```python
from build123d import *

# Parameters (mm, degrees)
SKETCH1_W           = 20
SKETCH1_H           = 25
SKETCH1_R           = 1
SKETCH1_W_2         = 12
SKETCH1_H_2         = 15
BOSS_EXTRUDE1_DEPTH = 1.5


with BuildPart() as part:
    # Sketch1 → Boss-Extrude1 (new, symmetric)
    with BuildSketch(Plane(origin=(0, 0, 0), x_dir=(1, 0, 0), z_dir=(0, 1, 0))):
        Rectangle(SKETCH1_W, SKETCH1_H)
        with Locations(Location((-8, -2.5, 0), (0, 0, 270))):
            Circle(SKETCH1_R, mode=Mode.SUBTRACT)
        with Locations(Location((8, -2.5, 0), (0, 0, 90))):
            Circle(SKETCH1_R, mode=Mode.SUBTRACT)
        Rectangle(SKETCH1_W_2, SKETCH1_H_2, mode=Mode.SUBTRACT)
    extrude(amount=BOSS_EXTRUDE1_DEPTH, both=True)


solid = part.part
```
CAD build for the part. Positions are in the model's coordinates, mm. A direction names the side the tool comes from. Coordinates: 2 decimals unless noted, no trailing zeros. Order: outer loops, then holes, each group sorted by start corner. A loop starts at its lowest first (then second) coordinate and runs counter-clockwise, first axis right, second up. Notation, with made-up numbers: (7, 3.25) - (35, 3.25) arc R22 cw to (35, 19.25) - close; hole circle Ø11 at (8.5, -33.5). An arc over 180 degrees is marked (long way). Answer in a Markdown table with one row per item.
1. Pull direction Z, two halves, no side cores. Call faces 1 (the face through (-7, 1.5, 0)), 2 (the face through (-6, 0, 0)), 3 (the face through (0, 0, 12.5)): +Z half, -Z half, draft (parallel to the pull), parting line (faces both ways), or undercut.
Answer:
| item | result |
|---|---|
| face 1 | draft |
| face 2 | undercut |
| face 3 | +Z half |
2. Drill centre lines: L1, parallel to X at y = -0.2, z = 2.5; L2, parallel to X at y = -0.3, z = -4.25; L3, parallel to Z at x = 5.75, y = -0.95. Where is each one in solid material? Low to high. Write a range as from..to.
Answer:
| item | result |
|---|---|
| L1 | -10..-9, -7..-6, 6..7, 9..10 |
| L2 | -10..-6, 6..10 |
| L3 | -12.5..-7.5, 7.5..12.5 |
3. 3-axis set-ups, long thin cutter, end or side, ignore diameter. For faces 4 (the face through (-7, -1.5, 0)), 5 (the face through (0, 0, 7.5)): which of +Z, -Z, +X, -X, +Y, -Y reach the whole face in a straight line?
Answer:
| item | result |
|---|---|
| face 4 | +Z, -Z, +X, -X, -Y |
| face 5 | +Y, -Y |
4. Slice it at B-B, the plane z = -2.5. List the corners of the cut face in (x, y), then the cut area to 3 significant figures.
Answer:
| item | result |
|---|---|
| outline | (-10, -1.5) - (-6, -1.5) - (-6, 1.5) - (-10, 1.5) - close; (6, -1.5) - (10, -1.5) - (10, 1.5) - (6, 1.5) - close |
| area | 24.0 mm² |
5. Slice it at C-C, the plane z = 2.5. List the corners of the cut face in (x, y).
Answer:
| item | result |
|---|---|
| outline | (-10, -1.5) - (-9, -1.5) - (-9, 1.5) - (-10, 1.5) - close; (-7, -1.5) - (-6, -1.5) - (-6, 1.5) - (-7, 1.5) - close; (6, -1.5) - (7, -1.5) - (7, 1.5) - (6, 1.5) - close; (9, -1.5) - (10, -1.5) - (10, 1.5) - (9, 1.5) - close |
6. Slice it at A-A, the plane x = -8. List the corners of the cut face in (y, z).
Answer:
| item | result |
|---|---|
| outline | (-1.5, -12.5) - (1.5, -12.5) - (1.5, 1.5) - (-1.5, 1.5) - close; (-1.5, 3.5) - (1.5, 3.5) - (1.5, 12.5) - (-1.5, 12.5) - close |
7. Slice it at D-D, the plane y = 0.2. List the corners of the cut face in (x, z), then the cut area to 3 significant figures.
Answer:
| item | result |
|---|---|
| outline | (-10, -12.5) - (10, -12.5) - (10, 12.5) - (-10, 12.5) - close; hole circle Ø2 at (-8, 2.5); hole (-6, -7.5) - (6, -7.5) - (6, 7.5) - (-6, 7.5) - close; hole circle Ø2 at (8, 2.5) |
| area | 314 mm² |
